Autodesk Inventor part; units mm, degrees
ref_plane "YZ Plane" through (0, 0, 0) normal (1, 0, 0) x (0, 1, 0)
ref_plane "XZ Plane" through (0, 0, 0) normal (0, 1, 0) x (-1, 0, 0)
ref_plane "XY Plane" through (0, 0, 0) normal (0, 0, 1) x (1, 0, 0)
sketch "Sketch5" plane through (0, 0, 0) normal (0, 0, 1) x (1, 0, 0)
  line L0 (-50, -8.5) -> (50, -8.5)
  line L1 (50, 8.5) -> (50, -8.5)
  line L2 (-50, 8.5) -> (50, 8.5)
  line L3 (-50, 8.5) -> (-50, -8.5)
  point P0 (0, 0)
  point P1 (0, 8.5)
  point P2 (50, 0)
  dimension "d8" = 100
  dimension "d9" = 17
extrude "Extrusion5" add sketch "Sketch5" along normal mid plane 62.5
chamfer "Chamfer1" distance 2 angle 45 2 edges at (50, -8.5, 0) (-50, -8.5, 0)
sketch "Sketch7" plane through (-48, -8.5, -31.25) normal (0, -1, 0) x (1, 0, 0)
  circle A0 centre (78, 15.75) radius 2.2423
  circle A1 centre (78, 46.75) radius 2.2423
  circle A2 centre (18, 15.75) radius 2.2423
  circle A3 centre (18, 46.75) radius 2.2423
  point P0 (48, 31.25)
  point P1 (96, 0)
  point P2 (96, 62.5)
  dimension "d18" = 60
  dimension "d19" = 30
  dimension "d20" = 31
  dimension "d21" = 15.5
  dimension "d48" = 62.5
hole "Hole1" at (30, -8.5, -15.5) at (30, -8.5, 15.5) at (-30, -8.5, 15.5) at (-30, -8.5, -15.5) direction (0, 1, 0) diameter 4.5 end through all counterbore diameter 8 counterbore depth 4.5
sketch "Sketch9" plane through (-48, -8.5, -31.25) normal (0, -1, 0) x (1, 0, 0)
  circle A0 centre (78, 15.75) radius 4
  circle A1 centre (78, 46.75) radius 4
  circle A2 centre (68, 46.75) radius 2.5
  circle A3 centre (68, 15.75) radius 2.5
  line L0 (48, 31.25) -> (48, 8.9232)
  circle A4 centre (28, 46.75) radius 2.5
  circle A5 centre (28, 15.75) radius 2.5
  dimension "d39" = 20
  dimension "d40" = 5
hole "Hole3" at (-20, -8.5, -15.5) at (-20, -8.5, 15.5) at (20, -8.5, 15.5) at (20, -8.5, -15.5) direction (0, 1, 0) diameter 4.134 end through all
chamfer "Chamfer4" distance 0.5 angle 45 14 edges at (0, 8.5, 31.25) (50, 8.5, 0) (-50, 8.5, 0) (0, 8.5, -31.25) (50, 1, 31.25) (50, 1, -31.25) (-50, 1, -31.25) (-50, 1, 31.25) (0, -8.5, 31.25) (0, -8.5, -31.25) (49, -7.5, 31.25) (-49, -7.5, 31.25) (49, -7.5, -31.25) (-49, -7.5, -31.25)
properties part number "BC-10022" material "Aço Carbono AISI 1006"
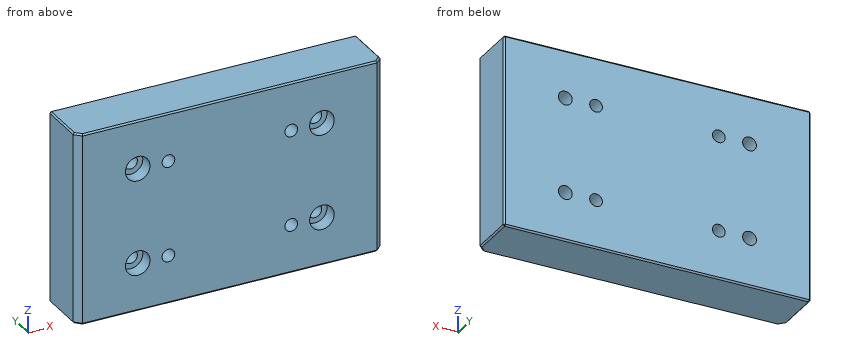
Read the model definition and answer for the solid it produces. Units are mm, in the model's axes. Give positions to 0.01 mm unless a question says otherwise; leave off trailing zeros. Loops run counter-clockwise (first coordinate to the right, second up) from the corner with the lowest first, then second, coordinate; pieces in that order, holes last.
Item 1: The part is cut by section A-A (x = 20). Write down the section's boundary in (y, z).
Item 2: The part is cut by section B-B (z = -15.5). Give the number of separate pieces and of enclosed holes in the cut face, and give its area (3 significant figures).
Item 3: Find the intervals of material crossed by line 1 along X through (y, z) = (-5, -15.5); line 2 along Z through (x, y) = (-20, 4); line 3 along X through (y, z) = (1.25, -15.5), in increasing order.
Item 4: The part is cut by section D-D (x = 30). Write down the section's boundary in (y, z), and give its area (4 significant figures).
Item 5: Each of these flat-tipped pins is pushed along its axis until it touches: pin 1 Ø4 at (x, z) = (30, 15.5) entering from -Y; pin 2 Ø5 at (x, z) = (-30, 15.5) entering from -Y. Where does it stop, or does it pass through?
Taken from the geometry:
1. outline: (-8.5, -30.75) - (-8, -31.25) - (8, -31.25) - (8.5, -30.75) - (8.5, -17.57) - (-8.5, -17.57) - close; (-8.5, -13.43) - (8.5, -13.43) - (8.5, 13.43) - (-8.5, 13.43) - close; (-8.5, 17.57) - (8.5, 17.57) - (8.5, 30.75) - (8, 31.25) - (-8, 31.25) - (-8.5, 30.75) - close
2. separate pieces: 5
2. enclosed holes: 0
2. area: 1,370 mm2
3. line 1: x = -50 to -34, -26 to -22.07, -17.93 to 17.93, 22.07 to 26, 34 to 50
3. line 2: z = -31.25 to -17.57, -13.43 to 13.43, 17.57 to 31.25
3. line 3: x = -50 to -32.25, -27.75 to -22.07, -17.93 to 17.93, 22.07 to 27.75, 32.25 to 50
4. outline: (-8.5, -30.75) - (-8, -31.25) - (8, -31.25) - (8.5, -30.75) - (8.5, -17.75) - (-4, -17.75) - (-4, -19.5) - (-8.5, -19.5) - close; (-8.5, -11.5) - (-4, -11.5) - (-4, -13.25) - (8.5, -13.25) - (8.5, 13.25) - (-4, 13.25) - (-4, 11.5) - (-8.5, 11.5) - close; (-8.5, 19.5) - (-4, 19.5) - (-4, 17.75) - (8.5, 17.75) - (8.5, 30.75) - (8, 31.25) - (-8, 31.25) - (-8.5, 30.75) - close
4. area: 877.5 mm2
5. pin 1: passes through
5. pin 2: stops at y = -4
